Verification items for the finished model (mm, model axes). A direction names the side the tool comes from. Give positions to 0.01 mm unless a question says otherwise; leave off trailing zeros. Write each loop counter-clockwise with the first axis right and the second up, starting at its lowest first coordinate (ties: lowest second). Pieces come first, ordered by that corner, then holes.
Autodesk Inventor part; units mm, degrees
ref_plane "Arbeitsebene1" through (0, 0, 15) normal (0, 0, 1) x (1, 0, 0)
ref_plane "YZ Plane" through (0, 0, 0) normal (1, 0, 0) x (0, 1, 0)
ref_plane "XZ Plane" through (0, 0, 0) normal (0, 1, 0) x (-1, 0, 0)
sketch "Skizze1" plane through (0, 0, 0) normal (0, 0, 1) x (1, 0, 0)
  line L0 (-110, -40) -> (110, -40)
  line L1 (110, -40) -> (110, 40)
  line L2 (110, 40) -> (-110, 40)
  line L3 (-110, 40) -> (-110, -40)
extrude "Extrusion1" add sketch "Skizze1" along normal blind 15
ref_plane "Arbeitsebene1" through (0, 0, 15) normal (0, 0, 1) x (1, 0, 0)
sketch "Skizze2" plane through (0, 0, 15) normal (0, 0, 1) x (1, 0, 0)
  line L0 (-83.25, -10.25) -> (-52.75, -10.25)
  line L1 (-52.75, -10.25) -> (-52.75, 10.25)
  line L2 (-52.75, 10.25) -> (-83.25, 10.25)
  line L3 (-83.25, 10.25) -> (-83.25, -10.25)
extrude "Extrusion2" cut sketch "Skizze2" against normal blind 2
sketch "Skizze3" plane through (0, 0, 15) normal (0, 0, 1) x (1, 0, 0)
  line L0 (52.75, -10.25) -> (83.25, -10.25)
  line L1 (83.25, -10.25) -> (83.25, 10.25)
  line L2 (83.25, 10.25) -> (52.75, 10.25)
  line L3 (52.75, 10.25) -> (52.75, -10.25)
extrude "Extrusion3" cut sketch "Skizze3" against normal blind 2
sketch "Skizze4" plane through (0, 0, 15) normal (0, 0, 1) x (1, 0, 0)
  line L0 (-53.25, -6.25) -> (53.25, -6.25)
  line L1 (53.25, -6.25) -> (53.25, 6.25)
  line L2 (53.25, 6.25) -> (-53.25, 6.25)
  line L3 (-53.25, 6.25) -> (-53.25, -6.25)
extrude "Extrusion4" cut sketch "Skizze4" against normal blind 2
sketch "Skizze5" plane through (0, 0, 15) normal (0, 0, 1) x (1, 0, 0)
  line L0 (-30, -25) -> (30, -25)
  line L1 (30, -25) -> (30, 25)
  line L2 (30, 25) -> (-30, 25)
  line L3 (-30, 25) -> (-30, -25)
extrude "Extrusion5" cut sketch "Skizze5" against normal blind 16
sketch "Skizze6" plane through (0, 0, 15) normal (0, 0, 1) x (1, 0, 0)
  circle A0 centre (-68, -15) radius 1.6
  circle A1 centre (-68, 15) radius 1.6
  circle A2 centre (68, -15) radius 1.6
  circle A3 centre (68, 15) radius 1.6
extrude "Extrusion6" cut sketch "Skizze6" against normal blind 16
properties part number "Grundplatte_v2"
Item 1: Sectioned sample at B-B on x = 3. Record the cut outline in (y, z).
Answer key:
outline: (-40, 0) - (-25, 0) - (-25, 15) - (-40, 15) - close; (25, 0) - (40, 0) - (40, 15) - (25, 15) - close
Item 2: Scan lines: line 1 along Y through (x, z) = (-68, 4.75); line 2 along Y through (x, z) = (-21, 1.25); line 3 along X through (y, z) = (16, 3.25). Record each from-to range of solid material in increasing order.
Answer key:
line 1: y = -40 to -16.6, -13.4 to 13.4, 16.6 to 40
line 2: y = -40 to -25, 25 to 40
line 3: x = -110 to -69.25, -66.75 to -30, 30 to 66.75, 69.25 to 110
Item 3: Set-up check for faces 5 (the face through (2, 40, 7)), 6 (the face through (0, 25, 8)): record each of +Z, -Z, +X, -X, +Y, -Y from which the full face is reachable in a straight line by a thin tool's end or side.
Answer key:
face 5: +Z, -Z, +X, -X, +Y
face 6: +Z, -Z
Item 4: Sectioned sample at A-A on y = 3.5. Record the cut outline in (x, z).
Answer key:
outline: (-110, 0) - (-30, 0) - (-30, 13) - (-83.25, 13) - (-83.25, 15) - (-110, 15) - close; (30, 0) - (110, 0) - (110, 15) - (83.25, 15) - (83.25, 13) - (30, 13) - close
Item 5: Release check for a two-part mould opening along X. For faces 1 (the face through (-110, 1, 7)), 2 (the face through (30, 0, 8)), 3 (the face through (-2, 27, 15)), 4 (the face through (0, -25, 8)) record: released by +X, released by -X, zero draft, split by the parting line, or undercut.
Answer key:
face 1: released by -X
face 2: undercut
face 3: zero draft
face 4: undercut
Item 6: Sectioned sample at C-C on z = 7.75. Record the cut outline in (x, y).
Answer key:
outline: (-110, -40) - (110, -40) - (110, 40) - (-110, 40) - close; hole circle Ø3.2 at (-68, -15); hole circle Ø3.2 at (-68, 15); hole (-30, -25) - (30, -25) - (30, 25) - (-30, 25) - close; hole circle Ø3.2 at (68, -15); hole circle Ø3.2 at (68, 15)
Item 7: Depth check by flat-ended pin: pin 1 (3.5 mm diameter, centred on x = -68, y = 15, fed in from +Z); pin 2 (6 mm diameter, centred on x = 60, y = -0.5, fed in from +Z). Enter the tip coordinate at first touch or a pass-through.
Answer key:
pin 1: stops at z = 15
pin 2: stops at z = 13
Item 8: Sectioned sample at D-D on x = 64. Record the cut outline in (y, z), then the cut area to 3 significant figures.
Answer key:
outline: (-40, 0) - (40, 0) - (40, 15) - (10.25, 15) - (10.25, 13) - (-10.25, 13) - (-10.25, 15) - (-40, 15) - close
area: 1,160 mm2
